from build123d import *

# Parameters (mm, degrees)
F1_DEPTH  = 7
F2_W      = 4
F2_H      = 12
F3_DEPTH  = 8
F4_W      = 12.2146774828
F4_H      = 1.6385169476
F5_DEPTH  = 8
F7_DEPTH  = 80
F8_R      = 2.25
F9_DEPTH  = 25
F10_W     = 40
F10_H     = 30
F10_R     = 2.25
F11_DEPTH = 4
F12_R     = 3
F14_DEPTH = 4
F15_W     = 15
F15_H     = 11.3999997266
F16_DEPTH = 4


with BuildPart() as f1:
    # F0 (on Top) → F1 (new body)
    with BuildSketch(Plane.XY):
        Polygon((-29, 15), (-33, 15), (-33, -1), (-45, -1), (-45, -15), (45, -15), (45, 15), (29, 15), align=None)
        with BuildLine():
            ThreePointArc((-28.25, 10), (-29.5303300859, 9.4696699141), (-29, 10.75))
            ThreePointArc((-29, 10.75), (-28.4696699141, 10.5303300859), (-28.25, 10))
        make_face(mode=Mode.SUBTRACT)
        with BuildLine():
            ThreePointArc((29.75, 10), (28.4696699141, 9.4696699141), (29, 10.75))
            ThreePointArc((29, 10.75), (29.5303300859, 10.5303300859), (29.75, 10))
        make_face(mode=Mode.SUBTRACT)
    extrude(amount=F1_DEPTH)

    # F2 (on face) → F3 (join)
    with BuildSketch(Plane.XY.offset(7)):
        Polygon((-33, -1), (-45, -1), (-45, -15), (-32.7853225172, -15), (-32.7853225172, -1), align=None)
        with Locations((43, -9)):
            Rectangle(F2_W, F2_H)
    extrude(amount=F3_DEPTH)

    # F4 (on face) → F5 (cut)
    with BuildSketch(Plane.XY.offset(15)):
        with Locations((-38.8926612586, -1.8192584738)):
            Rectangle(F4_W, F4_H)
    extrude(amount=-F5_DEPTH, mode=Mode.SUBTRACT)

    # F6 (on face) → F7 (cut)
    with BuildSketch(Plane.YZ.offset(45)):
        with BuildLine():
            ThreePointArc((-12.5, 9.4), (-11.3686291501, 9.8686291501), (-10.9, 11))
            ThreePointArc((-10.9, 11), (-13.6313708499, 12.1313708499), (-12.5, 9.4))
        make_face()
    extrude(amount=-F7_DEPTH, mode=Mode.SUBTRACT)

    # F8 (on face) → F9 (cut)
    with BuildSketch(Plane.XY.offset(7)):
        with Locations((-10, 0)):
            Circle(F8_R)
        with BuildLine():
            ThreePointArc((12.25, 0), (10, 2.25), (7.75, 0))
            ThreePointArc((7.75, 0), (10, -2.25), (12.25, 0))
        make_face()
    extrude(amount=-F9_DEPTH, mode=Mode.SUBTRACT)

    # F10 (on face) → F11 (cut)
    with BuildSketch(Plane.XY.offset(7)):
        Rectangle(F10_W, F10_H)
        with Locations((-10, 0)):
            Circle(F10_R, mode=Mode.SUBTRACT)
        with Locations((10, 0)):
            Circle(F10_R, mode=Mode.SUBTRACT)
    extrude(amount=-F11_DEPTH, mode=Mode.SUBTRACT)

    # F12
    f12_edges = [f1.edges().sort_by_distance(p)[0] for p in [
        (-38.892661, -15, 15),
        (43, -15, 15),
        (-38.892661, -2.638517, 15),
        (43, -3, 15),
    ]]
    fillet(f12_edges, radius=F12_R)

    # F13 (on Top) → F14 (join)
    with BuildSketch(Plane.XY):
        with BuildLine():
            Line((57.5766451657, 15.0159569457), (51.0659832507, 15.0159569457))
            Line((51.0659832507, 15.0159569457), (51.0659832507, 10.2579784729))
            ThreePointArc((51.0659832507, 10.2579784729), (53.010526899, 9.4525221211), (53.8159832507, 7.5079784729))
            ThreePointArc((53.8159832507, 7.5079784729), (53.010526899, 5.5634348246), (51.0659832507, 4.7579784729))
            Line((51.0659832507, 4.7579784729), (51.0659832507, 0))
            Line((51.0659832507, 0), (51.0659832507, -4.7165443972))
            ThreePointArc((51.0659832507, -4.7165443972), (53.010526899, -5.5220007489), (53.8159832507, -7.4665443972))
            ThreePointArc((53.8159832507, -7.4665443972), (53.010526899, -9.4110880454), (51.0659832507, -10.2165443972))
            Line((51.0659832507, -10.2165443972), (51.0659832507, -14.9330887944))
            Line((51.0659832507, -14.9330887944), (57.5766451657, -14.9330887944))
            Line((57.5766451657, -14.9330887944), (57.5766451657, 15.0159569457))
        make_face()
        with BuildLine():
            Line((51.0659832507, 15.0159569457), (44.5553213358, 15.0159569457))
            Line((44.5553213358, 15.0159569457), (44.5553213358, -14.9330887944))
            Line((44.5553213358, -14.9330887944), (51.0659832507, -14.9330887944))
            Line((51.0659832507, -14.9330887944), (51.0659832507, -10.2165443972))
            ThreePointArc((51.0659832507, -10.2165443972), (48.3159832507, -7.4665443972), (51.0659832507, -4.7165443972))
            Line((51.0659832507, -4.7165443972), (51.0659832507, 0))
            Line((51.0659832507, 0), (51.0659832507, 4.7579784729))
            ThreePointArc((51.0659832507, 4.7579784729), (48.3159832507, 7.5079784729), (51.0659832507, 10.2579784729))
            Line((51.0659832507, 10.2579784729), (51.0659832507, 15.0159569457))
        make_face()
    extrude(amount=F14_DEPTH)

    # F15 (on Top) → F16 (join)
    with BuildSketch(Plane.XY):
        with Locations((-52.2000010312, -9.1500000563)):
            Rectangle(F15_W, F15_H)
    extrude(amount=F16_DEPTH)


solid = f1.part
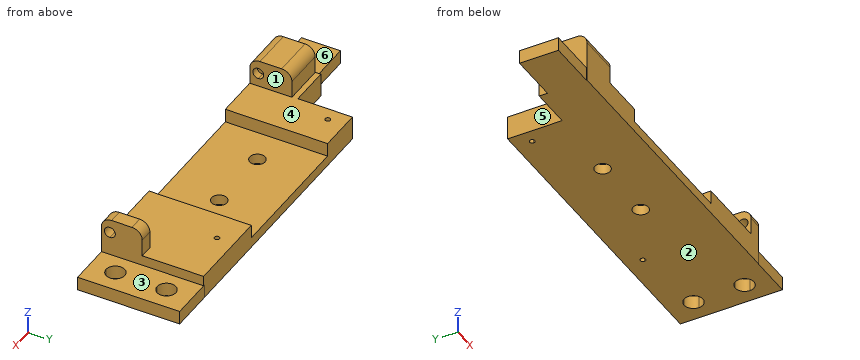
Check sheet for the modelled part. Datum: model origin and axes. Units: mm. Face numbers are marked on the shaded views. A direction names the side the tool comes from. Round coordinates to 2 decimals unless told otherwise and drop trailing zeros. Write each loop counter-clockwise with the first axis right and the second up, starting at its lowest first coordinate (ties: lowest second). Pieces come first, ordered by that corner, then holes. Notation, with made-up numbers: (40.5, 80.5) -> (73.5, 80.5) arc R28 ccw to (73.5, 102.5) -> close; hole circle Ø11 at (-28.5, 81.5). An arc over 180 degrees is marked (long way). Answer as CSV lines item,"result". Start each with the question number.
1) Section check D-D on y = 1. Enter the section's corners in (x, z), and give its area (3 significant figures).
2) Release check for a two-part mould opening along X. For the marked faces 4, 5 and 6 record: pulls with the +X half, pulls with the -X half, needs draft (parallel to the pull), parting line crosses it, or undercut.
3) Section check C-C on y = 6.5. Enter the section's corners in (x, z), and give its area (3 significant figures).
4) Go/stop test with flat-tipped pins: P1, Ø2, axis at x = -49.5, z = 1, coming from the +Y side; P2, Ø7, axis at x = 10, y = 0, coming from the +Z side; P3, Ø2, axis at x = 32, z = 4, coming from the +Y side. Record where each tip stops, or that it passes through.
5) Material ranges on line 1 (Y direction, x = 10, z = 0.65); line 2 (Y direction, x = 29, z = 1.5); line 3 (X direction, y = 7, z = 6.5), recorded low to high. Write a range as from..to.
6) Tool access check on the marked faces 1, 2 and 3. Record the directions out of +Z, -Z, +X, -X, +Y, -Y that give a thin tool (end or side, any length) a straight path to the whole face; none if there is none.
7) Section check A-A on z = 5.25. Enter the section's corners in (x, y), and give its area (3 significant figures).
8) Section check B-B on x = -10. Enter the section's corners in (y, z), and give its area (3 significant figures).
Found:
1,outline,"(-33, 0) -> (-12.02, 0) -> (-12.02, 3) -> (-20, 3) -> (-20, 7) -> (-33, 7) -> close; (-7.98, 0) -> (7.98, 0) -> (7.98, 3) -> (-7.98, 3) -> close; (12.02, 0) -> (57.58, 0) -> (57.58, 4) -> (45, 4) -> (45, 7) -> (20, 7) -> (20, 3) -> (12.02, 3) -> close"
1,area,"412 mm^2"
2,face 4,"undercut"
2,face 5,"pulls with the -X half"
2,face 6,"needs draft"
3,outline,"(-33, 0) -> (48.51, 0) -> (48.51, 4) -> (45, 4) -> (45, 7) -> (20, 7) -> (20, 3) -> (-20, 3) -> (-20, 7) -> (-33, 7) -> close; (53.62, 0) -> (57.58, 0) -> (57.58, 4) -> (53.62, 4) -> close"
3,area,"416 mm^2"
4,P1,"stops at y = -3.45"
4,P2,"stops at z = 3"
4,P3,"stops at y = 15"
5,line 1,"y = -15..-2.25, 2.25..15"
5,line 2,"y = -15..9.25, 10.75..15"
5,line 3,"x = -33..-20, 20..45"
6,face 1,"+Z, +Y, -Y"
6,face 2,"-Z, +X, -X, +Y, -Y"
6,face 3,"+Z, +X, +Y, -Y"
7,outline,"(-45, -15) -> (-20, -15) -> (-20, 15) -> (-33, 15) -> (-33, -1) -> (-45, -1) -> close; (20, -15) -> (45, -15) -> (45, 15) -> (20, 15) -> close; hole circle Ø1.5 at (-29, 10); hole circle Ø1.5 at (29, 10)"
7,area,"1,300 mm^2"
8,outline,"(-15, 0) -> (-2.25, 0) -> (-2.25, 3) -> (-15, 3) -> close; (2.25, 0) -> (15, 0) -> (15, 3) -> (2.25, 3) -> close"
8,area,"76.5 mm^2"
